Read the model definition and answer for the solid it produces. Units are mm, in the model's axes. A direction names the side the tool comes from. Coordinates: 2 decimals unless noted, no trailing zeros. Write each loop counter-clockwise with the first axis right and the second up, starting at its lowest first coordinate (ties: lowest second). Pieces come first, ordered by that corner, then holes.
(1) Straight lines are drawn through the part: line 1 along Y through (x, z) = (0, 0.65); line 2 along Y through (x, z) = (0, 0.4); line 3 along Z through (x, y) = (2.25, 2.5). For each, find the intervals that lie inside material, in ascending order.
(2) Determine the mould class of faces 1 (the cylindrical face through (0, -1, 1)), 2 (the flat face through (-1, -1, 0)), 3 (the cylindrical face through (-3.434, 1.081, 0.296)) for opening direction Y: pulls with the +Y half, pulls with the -Y half, needs draft (parallel to the pull), parting line crosses it, or undercut.
(3) The part is cut by section D-D, the plane x = -1.5. Determine the outline of the cut face in (y, z), and give its area (3 significant figures).
(4) The part is cut by section C-C, the plane z = 0.9. Determine the outline of the cut face in (x, y).
(5) Given pin 1 (1.2 mm diameter, centred on x = 0, y = 0, fed in from +Z), flat-ended and moving along its own axis, determine where the tip first touches the part or whether it passes through.
(6) Which of the six approach directions +Z, -Z, +X, -X, +Y, -Y give full straight-line access (tool end or side, diameter ignored) to faces 4 (the flat face through (-1, 1, 2)), 5 (the cylindrical face through (-3, 0, 1))?
(7) The part is cut by section A-A, the plane y = 0. Determine the outline of the cut face in (x, z).
```python
from build123d import *

# Parameters (mm, degrees)
SKETCH_1_R               = 3
EXTRUDE_1_DEPTH          = 2
SKETCH_3_R               = 3.6
EXTRUDE_2_DEPTH          = 0.6
SKETCH_4_R               = 1
CUT_EXTRUDE_1_DEPTH      = 1
CUT_EXTRUDE_1_DEPTH_BACK = 3


with BuildPart() as part:
    # Эскиз1 → Бобышка-Вытянуть1 (new body)
    with BuildSketch(Plane.XY):
        Circle(SKETCH_1_R)
    extrude(amount=EXTRUDE_1_DEPTH)

    # Эскиз3 → Бобышка-Вытянуть2 (add)
    with BuildSketch(Plane(origin=(0, 0, 0), x_dir=(-1, 0, 0), z_dir=(0, 0, -1))):
        Circle(SKETCH_3_R)
    extrude(amount=-EXTRUDE_2_DEPTH)

    # Эскиз4 → Вырез-Вытянуть1 (cut, two sides)
    with BuildSketch(Plane.XY.offset(2)) as cut_extrude_1_sk:
        Circle(SKETCH_4_R)
    extrude(amount=CUT_EXTRUDE_1_DEPTH, mode=Mode.SUBTRACT)
    extrude(cut_extrude_1_sk.sketch, amount=-CUT_EXTRUDE_1_DEPTH_BACK, mode=Mode.SUBTRACT)


solid = part.part
```
Computed:
1. line 1: y = -3 to -1, 1 to 3
1. line 2: y = -3.6 to -1, 1 to 3.6
1. line 3: z = 0 to 0.6
2. face 1: undercut
2. face 2: needs draft
2. face 3: parting line crosses it
3. outline: (-3.27, 0) - (3.27, 0) - (3.27, 0.6) - (2.6, 0.6) - (2.6, 2) - (-2.6, 2) - (-2.6, 0.6) - (-3.27, 0.6) - close
3. area: 11.2 mm2
4. outline: circle Ø6 at (0, 0); hole circle Ø2 at (0, 0)
5. pin 1: passes through
6. face 4: +Z, +X, -X, +Y, -Y
6. face 5: +Z
7. outline: (-3.6, 0) - (-1, 0) - (-1, 2) - (-3, 2) - (-3, 0.6) - (-3.6, 0.6) - close; (1, 0) - (3.6, 0) - (3.6, 0.6) - (3, 0.6) - (3, 2) - (1, 2) - close
